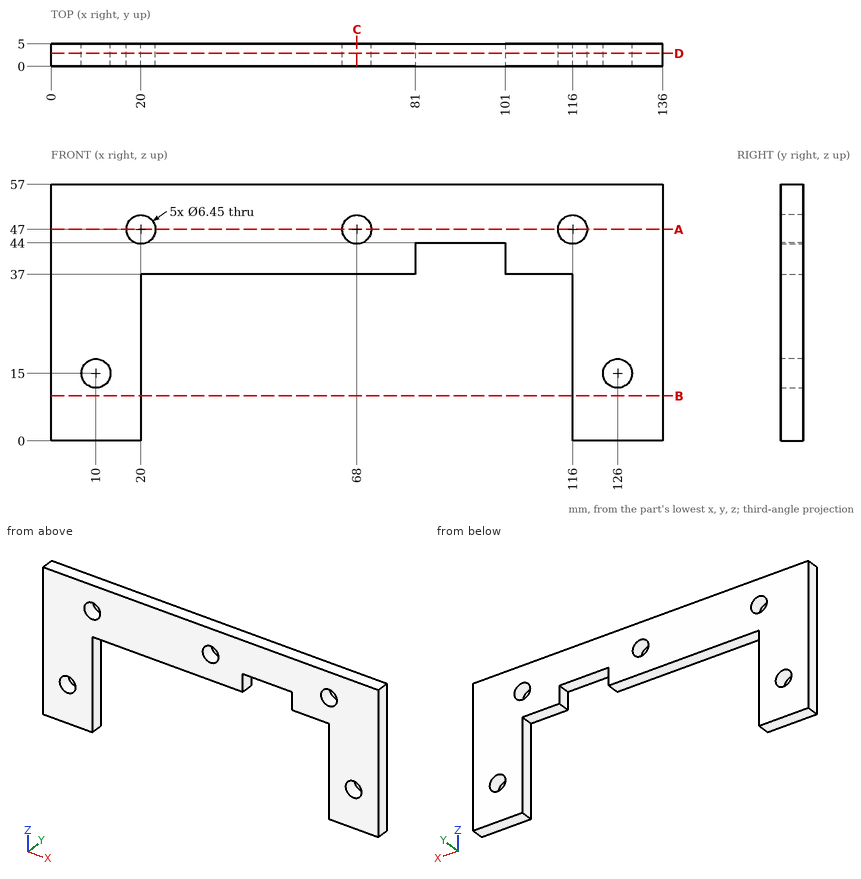
Job drawing, mm, ordinate dimensions from the low corner. One solid piece. Round coordinates to 2 decimals unless told otherwise and drop trailing zeros. Loops run counter-clockwise (first coordinate to the right, second up) from the corner with the lowest first, then second, coordinate; pieces in that order, holes last.
(1) Wall check: line 1 along X through (y, z) = (3.1, 15) (3 decimals); line 2 along X through (y, z) = (3.15, 47) (3 decimals); line 3 along X through (y, z) = (2.3, 33.5). Give the ranges that are in metal, low to high.
(2) Cut at B-B (z = 10). Give the cut face in (x, y), plus the area to 3 significant figures.
(3) Drop a flat-ended pin along its axis: pin 1 (1.5 mm diameter, centred on x = 69, y = 0.5, fed in from -Z). Give the stop position or say it passes through.
(4) Cut at C-C (x = 68). Give the cut face in (y, z) (3 decimals).
(5) Cut at D-D (y = 2.9). Give the cut face in (x, z) (3 decimals), plus the area to 3 significant figures.
(6) Cut at A-A (z = 47). Give the cut face in (x, y) (3 decimals), plus the area to 3 significant figures.
Findings below:
1. line 1: x = 0 to 6.775, 13.225 to 20, 116 to 122.775, 129.225 to 136
1. line 2: x = 0 to 16.775, 23.225 to 64.775, 71.225 to 112.775, 119.225 to 136
1. line 3: x = 0 to 20, 116 to 136
2. outline: (0, 0) - (20, 0) - (20, 5) - (0, 5) - close; (116, 0) - (136, 0) - (136, 5) - (116, 5) - close
2. area: 200 mm2
3. pin 1: stops at z = 37
4. outline: (0, 37) - (5, 37) - (5, 43.775) - (0, 43.775) - close; (0, 50.225) - (5, 50.225) - (5, 57) - (0, 57) - close
5. outline: (0, 0) - (20, 0) - (20, 37) - (81, 37) - (81, 44) - (101, 44) - (101, 37) - (116, 37) - (116, 0) - (136, 0) - (136, 57) - (0, 57) - close; hole circle Ø6.45 at (10, 15); hole circle Ø6.45 at (20, 47); hole circle Ø6.45 at (68, 47); hole circle Ø6.45 at (116, 47); hole circle Ø6.45 at (126, 15)
5. area: 3,900 mm2
6. outline: (0, 0) - (16.775, 0) - (16.775, 5) - (0, 5) - close; (23.225, 0) - (64.775, 0) - (64.775, 5) - (23.225, 5) - close; (71.225, 0) - (112.775, 0) - (112.775, 5) - (71.225, 5) - close; (119.225, 0) - (136, 0) - (136, 5) - (119.225, 5) - close
6. area: 583 mm2
